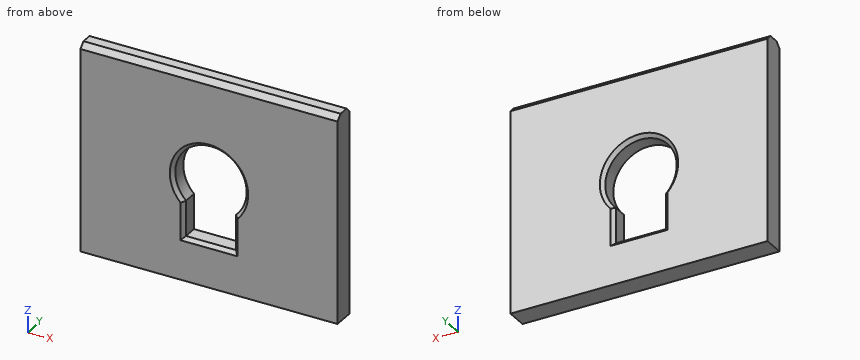
```python
from build123d import *

# Parameters (mm, degrees)
F0_W     = 73.423766
F0_H     = 59.146922
F1_DEPTH = 6
F2_SIZE  = 1
F3_SIZE  = 1.5


with BuildPart() as f1:
    # F0 (on Front) → F1 (new body)
    with BuildSketch(Plane.XZ):
        Rectangle(F0_W, F0_H)
        with BuildLine():
            Line((7.138422, -7.285804), (7.138422, -17.335804))
            Line((7.138422, -17.335804), (-7.138422, -17.335804))
            Line((-7.138422, -17.335804), (-7.138422, -7.285804))
            ThreePointArc((-7.138422, -7.285804), (0, 10.2), (7.138422, -7.285804))
        make_face(mode=Mode.SUBTRACT)
    extrude(amount=F1_DEPTH)

    # F2
    f2_edges = [f1.edges().sort_by_distance(p)[0] for p in [
        (0, -6, 10.2),
        (-7.138422, -6, -12.310804),
        (0, -6, -17.335804),
        (7.138422, -6, -12.310804),
        (0, 0, -17.335804),
        (-7.138422, 0, -12.310804),
        (0, 0, 10.2),
        (7.138422, 0, -12.310804),
    ]]
    chamfer(f2_edges, length=F2_SIZE)

    # F3
    f3_edges = [f1.edges().sort_by_distance(p)[0] for p in [
        (0, -6, 29.573461),
        (0, 0, 29.573461),
    ]]
    chamfer(f3_edges, length=F3_SIZE)


solid = f1.part
```
Read the model definition and answer for the solid it produces. Units are mm, in the model's axes. Coordinates: 2 decimals unless noted, no trailing zeros. Order: outer loops, then holes, each group sorted by start corner. A loop starts at its lowest first (then second) coordinate and runs counter-clockwise, first axis right, second up. Notation, with made-up numbers: (-0.75, 29.5) - (42.25, 29.5) arc R23 ccw to (42.25, 52.5) - close; hole circle Ø7 at (47.25, -24). An arc over 180 degrees is marked (long way). Answer as a JSON object with one key per item and string values. Group by question number.
Item 1: Section C-C (y = -3) is taken. Give the vertices of the cut face in (x, z), plus the area to 3 significant figures.
Item 2: Section A-A (z = 0) is taken. Give the vertices of the cut face in (x, y), plus the area to 3 significant figures.
Item 3: Consider probe 1 along Z at (x, y) = (0, -2.95); probe 2 along X at (y, z) = (-3.7, 0); probe 3 along X at (y, z) = (-3.75, -15.5). Determine where each line is inside the solid, lowest interval first. Write a range as from..to.
Item 4: Section B-B (x = 0) is taken. Give the vertices of the cut face in (y, z).
Item 5: Section D-D (z = -14.5) is taken. Give the vertices of the cut face in (x, y), plus the area to 3 significant figures.
Results are:
{
 "1": {"outline": "(-36.71, -29.57) - (36.71, -29.57) - (36.71, 29.57) - (-36.71, 29.57) - close; hole (-7.14, -17.34) - (7.14, -17.34) - (7.14, -7.29) arc R10.2 ccw (long way) to (-7.14, -7.29) - close", "area": "3,900 mm^2"},
 "2": {"outline": "(-36.71, -6) - (-11.2, -6) - (-10.2, -5) - (-10.2, -1) - (-11.2, 0) - (-36.71, 0) - close; (10.2, -5) - (11.2, -6) - (36.71, -6) - (36.71, 0) - (11.2, 0) - (10.2, -1) - close", "area": "316 mm^2"},
 "3": {"probe 1": "z = -29.57..-17.34, 10.2..29.57", "probe 2": "x = -36.71..-10.2, 10.2..36.71", "probe 3": "x = -36.71..-7.14, 7.14..36.71"},
 "4": {"outline": "(-6, -29.57) - (0, -29.57) - (0, -18.34) - (-1, -17.34) - (-5, -17.34) - (-6, -18.34) - close; (-6, 11.2) - (-5, 10.2) - (-1, 10.2) - (0, 11.2) - (0, 28.07) - (-1.5, 29.57) - (-4.5, 29.57) - (-6, 28.07) - close"},
 "5": {"outline": "(-36.71, -6) - (-8.14, -6) - (-7.14, -5) - (-7.14, -1) - (-8.14, 0) - (-36.71, 0) - close; (7.14, -5) - (8.14, -6) - (36.71, -6) - (36.71, 0) - (8.14, 0) - (7.14, -1) - close", "area": "353 mm^2"}
}
